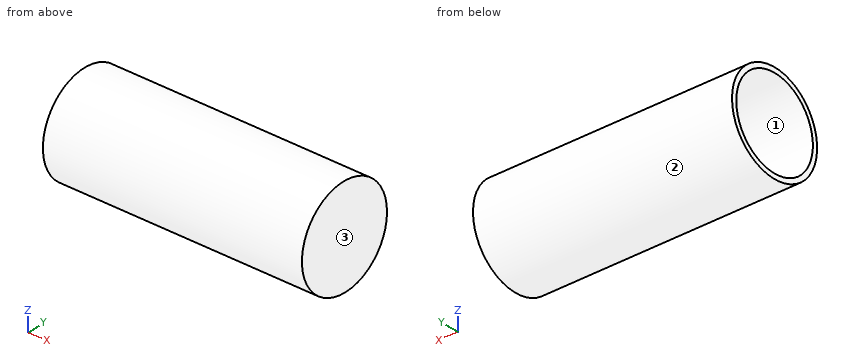
```python
from build123d import *

# Parameters (mm, degrees)
CUT_EXTRUDE1_START  = -0.5
CUT_EXTRUDE1_DEPTH  = 2
CIRPATTERN1_COUNT   = 8
SKETCH3_R           = 0.75
SKETCH3_R_2         = 0.625
BOSS_EXTRUDE1_DEPTH = 2.5


with BuildPart() as part:
    # Sketch1 → Revolve1 (revolve)
    with BuildSketch(Plane.XY):
        Polygon((0, 0), (0, 1), (-1, 2), (-7, 2), (-7, 4), (-10, 4), (-10, 3), (-13, 3), (-14.5, 4.5), (-24.88, 4.5), (-24.88, 5), (1.5, 5), (1.5, 0), align=None)
    revolve(axis=Axis((1.5, 0, 0), (-1, 0, 0)))

    # Sketch2 → Cut-Extrude1 (cut)
    with BuildSketch(Plane.ZY.offset(7).offset(CUT_EXTRUDE1_START)):
        with BuildLine():
            Line((-2, -0.1), (-3.9, -0.1))
            ThreePointArc((-3.9, -0.1), (-4, 0), (-3.9, 0.1))
            Line((-3.9, 0.1), (-2, 0.1))
            ThreePointArc((-2, 0.1), (-1.9, 0), (-2, -0.1))
        make_face()
    cut_extrude1 = extrude(amount=CUT_EXTRUDE1_DEPTH, mode=Mode.SUBTRACT)

    # CirPattern1: Cut-Extrude1 ×8 about axis
    cirpattern1_axis = Axis((0, 0, 0), (1, 0, 0))
    for i in range(1, CIRPATTERN1_COUNT):
        add(cut_extrude1.rotate(cirpattern1_axis, i * 360 / CIRPATTERN1_COUNT), mode=Mode.SUBTRACT)

    # Sketch3 → Boss-Extrude1 (add)
    with BuildSketch(Plane.ZY):
        with Locations(Location((0, 0, 0), (0, 0, 270))):
            Circle(SKETCH3_R)
        with Locations(Location((0, 0, 0), (0, 0, 270))):
            Circle(SKETCH3_R_2, mode=Mode.SUBTRACT)
    extrude(amount=BOSS_EXTRUDE1_DEPTH)


solid = part.part
```
Design review of the part built by this model. Coordinates are the model's own, in mm. Face numbers are marked on the shaded views. Coordinates: 2 decimals unless noted, no trailing zeros. Write each loop counter-clockwise with the first axis right and the second up, starting at its lowest first coordinate (ties: lowest second). Pieces come first, ordered by that corner, then holes. Notation, with made-up numbers: M 59,56 L 68,56 A12 ccw 68,63 Z; hole C -40,-10.75 d4. An arc over 180 degrees is marked long. Answer as a JSON object with one key per item and string values.
Item 1: Add section A-A, the plane x = -22. Give the boundary of the cut face in (y, z).
Outcome:
{"outline": "C 0,0 d10; hole C 0,0 d9"}
Item 2: Draft analysis for pull direction Z (two halves, no side actions). For the marked faces 1, 2 and 3, state which applies: pulls with the +Z half, pulls with the -Z half, needs draft (parallel to the pull), parting line crosses it, or undercut.
Outcome:
{"face 1": "undercut", "face 2": "parting line crosses it", "face 3": "needs draft"}
Item 3: Add section B-B, the plane x = -10.5. Give the boundary of the cut face in (y, z).
Outcome:
{"outline": "C 0,0 d10; hole C 0,0 d6"}
Item 4: Wall thickness on probe 1 along Z at (x, y) = (-8.7, 0); probe 2 along Y at (x, z) = (-2.25, 0.5) (1 decimal): over which ranges is each line inside the solid? List them lowest first.
Outcome:
{"probe 1": "-5 to -4, 4 to 5", "probe 2": "-5 to -1.9, -0.6 to -0.4, 0.4 to 0.6, 1.9 to 5"}
Item 5: Insertion check: pin 1 Ø1.2 at (y, z) = (0, 0.5) entering from -X; pin 2 Ø1.3 at (y, z) = (1.5, 2.5) entering from -X; pin 3 Ø1.7 at (y, z) = (-2, -2) entering from -X. Each pin has a flat end and moves straight along its axis. Give the tip position at first contact, or say it passes through.
Outcome:
{"pin 1": "x = -2.5", "pin 2": "x = -13.57", "pin 3": "x = -13.68"}
